from build123d import *

# Parameters (mm, degrees)
F1_DEPTH = 63.5
F2_DEPTH = 25.4
F3_DEPTH = 7.9375
F0_W     = 39.053507328
F0_H     = 28.575
F5_R     = 5.08


with BuildPart() as f1:
    # F0 (on Front) → F1 (new body, symmetric)
    with BuildSketch(Plane.XZ):
        Polygon((-41.275, 9.525), (-41.275, -9.525), (41.275, -9.525), (41.275, 9.525), (22.225, 9.525), align=None)
    extrude(amount=F1_DEPTH, both=True)

    # F0 (on Front) → F2 (join, symmetric)
    with BuildSketch(Plane.XZ):
        with BuildLine():
            Line((22.225, 9.525), (41.275, 9.525))
            Line((41.275, 9.525), (41.275, 27.0002))
            ThreePointArc((41.275, 27.0002), (45.9246798487, 38.2255201513), (57.15, 42.8752))
            Line((57.15, 42.8752), (60.325, 42.8752))
            Line((60.325, 42.8752), (60.325, 61.9252))
            Line((60.325, 61.9252), (57.15, 61.9252))
            ThreePointArc((57.15, 61.9252), (32.4542956671, 51.6959043329), (22.225, 27.0002))
            Line((22.225, 27.0002), (22.225, 9.525))
        make_face()
        Polygon((60.325, 66.675), (60.325, 61.9252), (60.325, 42.8752), (60.325, 38.1), (72.071492672, 38.1), (72.071492672, 66.675), align=None)
    extrude(amount=F2_DEPTH, both=True)

    # F0 (on Front) → F3 (join, symmetric)
    with BuildSketch(Plane.XZ):
        with BuildLine():
            add(Edge.make_bspline(
                [(-41.275, 9.525), (-40.8343672752, 33.3350226283), (22.7826405317, 62.8510192037), (57.15, 61.9252)],
                knots=[0, 0, 0, 0, 111.5045361635, 111.5045361635, 111.5045361635, 111.5045361635], degree=3))
            Line((-41.275, 9.525), (22.225, 9.525))
            Line((22.225, 9.525), (22.225, 27.0002))
            ThreePointArc((22.225, 27.0002), (32.4542956671, 51.6959043329), (57.15, 61.9252))
        make_face()
    extrude(amount=F3_DEPTH, both=True)

    # F0 (on Front) → F4 (revolve)
    with BuildSketch(Plane.XZ):
        with Locations((91.598246336, 52.3875)):
            Rectangle(F0_W, F0_H)
    revolve(axis=Axis((72.071492672, 0, 52.3875), (0, 0, 1)))

    # F5
    f5_edges = [f1.edges().sort_by_distance(p)[0] for p in [
        (41.275, -63.5, 0),
        (41.275, 63.5, 0),
        (-41.275, 63.5, 0),
        (-41.275, -63.5, 0),
    ]]
    fillet(f5_edges, radius=F5_R)


solid = f1.part
The model under review builds one solid part; all positions refer to its coordinate system, in mm. A direction names the side the tool comes from. Coordinates: 2 decimals unless noted, no trailing zeros. Loops run counter-clockwise (first coordinate to the right, second up) from the corner with the lowest first, then second, coordinate; pieces in that order, holes last. Notation, with made-up numbers: M 18,-23.75 L 26,-23.75 A20 cw 26,15.25 Z; hole C 70.5,8.5 d4. An arc over 180 degrees is marked long. Put each result on its own line as item: value. Start each with the question number.
Q1. Add section B-B (y = -15). Write out the cut boundary in (x, z) (3 decimals).
Q2. Wall thickness on line 1 (Y direction, x = 14, z = 46); line 2 (X direction, y = -11, z = 12) (3 decimals); line 3 (Z direction, x = -34, y = 39.5) (3 decimals): over which ranges is each line inside the solid? List them lowest first.
Q3. Add section A-A (z = -3). Write out the cut boundary in (x, y) (3 decimals).
Q4. Add section C-C (x = 95.5). Write out the cut boundary in (y, z) (1 decimal), and give its area (3 significant figures).
Q5. Add section D-D (y = -49). Write out the cut boundary in (x, z) (3 decimals), and give its area (3 significant figures).
Q6. Clearance check with flat-ended pins moving along their axes: pin 1 (19 mm diameter, centred on x = 33.5, z = 41, fed in from +Y); pin 2 (11 mm diameter, centred on y = -22.5, z = 0.5, fed in from +X) (3 decimals); pin 3 (8 mm diameter, centred on x = 26, z = 22, fed in from -Y). State where each tip first meets the part, or that it passes through.
Q7. For faces 1 (the cylindrical face through (-39.8, 62, -0.1)), 2 (the flat face through (22.225, 17, 18)), 3 (the flat face through (-3, -7.938, 29)), list the 3-axis set-ups (+Z, -Z, +X, -X, +Y, -Y) from which the entire face can be reached by the end or side of a thin tool; tool diameter is ignored.
Answers:
1. outline: M -41.275,-9.525 L 41.275,-9.525 L 41.275,27 A15.875 cw 45.801,38.1 L 108.129,38.1 L 108.129,66.675 L 36.014,66.675 L 36.014,54.803 A34.925 ccw 22.225,27 L 22.225,9.525 L -41.275,9.525 Z
2. line 1: y = -7.94 to 7.94
2. line 2: x = 22.225 to 41.275
2. line 3: z = -9.525 to 9.525
3. outline: M -41.275,-58.42 A5.08 ccw -36.195,-63.5 L 36.195,-63.5 A5.08 ccw 41.275,-58.42 L 41.275,58.42 A5.08 ccw 36.195,63.5 L -36.195,63.5 A5.08 ccw -41.275,58.42 Z
4. outline: M -31.2,38.1 L 31.2,38.1 L 31.2,66.7 L -31.2,66.7 Z
4. area: 1,790 mm^2
5. outline: M -41.275,-9.525 L 41.275,-9.525 L 41.275,9.525 L -41.275,9.525 Z
5. area: 1,570 mm^2
6. pin 1: stops at y = 26.08
6. pin 2: stops at x = 41.275
6. pin 3: stops at y = -25.4
7. face 1: +Z, -Z, -X, +Y
7. face 2: +Z, -X, +Y
7. face 3: +Z, -X, -Y
